```python
from build123d import *

# Parameters (mm, degrees)
SKETCH1_W             = 22
SKETCH1_H             = 9
SKETCH1_R             = 3
BOSS_EXTRUDE1_DEPTH   = 10
FILLET1_R             = 5
M3_TAPPED_HOLE1_D     = 2.5
M3_TAPPED_HOLE1_DEPTH = 7.5
M3_TAPPED_HOLE1_TIP   = 0.751075774


with BuildPart() as part:
    # Sketch1 → Boss-Extrude1 (new body)
    with BuildSketch(Plane(origin=(0, 0, 0), x_dir=(0, 0, -1), z_dir=(1, 0, 0))):
        with Locations((5, -0.5)):
            Rectangle(SKETCH1_W, SKETCH1_H)
        Circle(SKETCH1_R, mode=Mode.SUBTRACT)
        with Locations((10, 0)):
            Circle(SKETCH1_R, mode=Mode.SUBTRACT)
    extrude(amount=BOSS_EXTRUDE1_DEPTH)

    # Fillet1
    fillet1_edges = [part.edges().sort_by_distance(p)[0] for p in [
        (5, -5, -16),
        (5, -5, 6),
    ]]
    fillet(fillet1_edges, radius=FILLET1_R)

    # M3 Tapped Hole1
    with Locations(Plane(origin=(0, 4, 0), x_dir=(1, 0, 0), z_dir=(0, 1, 0))):
        with Locations((5, 5)):
            Hole(M3_TAPPED_HOLE1_D / 2, depth=M3_TAPPED_HOLE1_DEPTH)
            with Locations((0, 0, -(M3_TAPPED_HOLE1_DEPTH + M3_TAPPED_HOLE1_TIP / 2))):  # 118° drill point
                Cone(0, M3_TAPPED_HOLE1_D / 2, M3_TAPPED_HOLE1_TIP, mode=Mode.SUBTRACT)


solid = part.part
```
Can you work these out from the model? Positions are in its coordinate system, mm. A direction names the side the tool comes from. Coordinates: 2 decimals unless noted, no trailing zeros. Loops run counter-clockwise (first coordinate to the right, second up) from the corner with the lowest first, then second, coordinate; pieces in that order, holes last. Notation, with made-up numbers: (1, -17.75) - (27, -17.75) arc R21 cw to (27, 6.25) - close; hole circle Ø3 at (69, -1). An arc over 180 degrees is marked (long way). Answer as CSV lines item,"result". Start each with the question number.
1) Suppose I cut it at D-D (y = 2.5). Please give me the cut outline in (x, z), plus the area to 3 significant figures.
2) Suppose I cut it at A-A (y = 0.5). Please give me the cut outline in (x, z), plus the area to 3 significant figures.
3) Suppose I cut it at B-B (z = -10). Please give me the cut outline in (x, y), plus the area to 3 significant figures.
4) Thinking about a two-plate mould opening in Z: for faces 1 (the cylindrical face through (5, 0, 3)), 2 (the cylindrical face through (4.93, -1.15, -12.77)), 3 (the flat face through (0, 0, -5)), 4 (the flat face through (5, 2, 6)), which applies, pulls with the +Z half, pulls with the -Z half, needs draft (parallel to the pull), parting line crosses it, or undercut?
5) I need wall thicknesses on line 1 (Y direction, x = 3.75, z = -10); line 2 (Z direction, x = 6, y = 2.75); line 3 (Z direction, x = 9.25, y = 1). Which ranges of each line are inside material? Lowest first, please. Write a range as from..to.
6) For pin 1 (2 mm diameter, centred on y = 2.5, z = -12.5, fed in from -X), with a flat end and sliding along its axis, tell me the tip position at first contact or that it passes through.
7) Suppose I cut it at C-C (x = 1.25). Please give me the cut outline in (y, z).
8) Which directions (+Z, -Z, +X, -X, +Y, -Y) give clear straight access to the entire face, cutting with the end or side of a thin tool? Please do faces 5 (the flat face through (3, 4, -5)), 6 (the cylindrical face through (5.27, 0.2, -3.78)).
Check result:
1,outline,"(0, -16) - (10, -16) - (10, -11.66) - (0, -11.66) - close; (0, -8.34) - (10, -8.34) - (10, -1.66) - (0, -1.66) - close; (0, 1.66) - (10, 1.66) - (10, 6) - (0, 6) - close; hole circle Ø2.5 at (5, -5)"
1,area,"149 mm²"
2,outline,"(0, -16) - (10, -16) - (10, -12.96) - (0, -12.96) - close; (0, -7.04) - (10, -7.04) - (10, -2.96) - (0, -2.96) - close; (0, 2.96) - (10, 2.96) - (10, 6) - (0, 6) - close; hole circle Ø2.5 at (5, -5)"
2,area,"96.8 mm²"
3,outline,"(0, -5) - (10, -5) - (10, -3) - (0, -3) - close; (0, 3) - (10, 3) - (10, 4) - (0, 4) - close"
3,area,"30.0 mm²"
4,face 1,"undercut"
4,face 2,"undercut"
4,face 3,"needs draft"
4,face 4,"pulls with the +Z half"
5,line 1,"y = -5..-3, 3..4"
5,line 2,"z = -16..-11.2, -8.8..-5.75, -4.25..-1.2, 1.2..6"
5,line 3,"z = -16..-12.83, -7.17..-2.83, 2.83..6"
6,pin 1,"stops at x = 0"
7,outline,"(-5, -11) arc R5 ccw to (0, -16) - (4, -16) - (4, 6) - (0, 6) arc R5 ccw to (-5, 1) - close; hole circle Ø6 at (0, -10); hole circle Ø6 at (0, 0)"
8,face 5,"+Z, -Z, +X, -X, +Y"
8,face 6,"+Y"
